Answer from the drawing. Dimensions are ordinates in mm from the lowest x, y and z of the part. A direction names the side the tool comes from. Give positions to 0.01 mm unless a question says otherwise; leave off trailing zeros. Loops run counter-clockwise (first coordinate to the right, second up) from the corner with the lowest first, then second, coordinate; pieces in that order, holes last. Notation, with made-up numbers: (16.5, 86) - (54.5, 86) arc R5 cw to (54.5, 92) - close; hole circle Ø2 at (-27, -14). An arc over 180 degrees is marked (long way). Answer as CSV lines item,"result". Start each with the question number.
1) A cutting plane is placed at D-D (z = 4.5). Determine the outline of the cut face in (x, y), and give its area (3 significant figures).
2) For a pull along X with two mould halves and no side action, classify the marked faces 3, 4, 5 and 6 as pulls with the +X half, pulls with the -X half, needs draft (parallel to the pull), parting line crosses it, or undercut.
3) A cutting plane is placed at B-B (x = 45.6). Determine the outline of the cut face in (y, z).
4) A cutting plane is placed at A-A (y = 21.4). Determine the outline of the cut face in (x, z).
5) A cutting plane is placed at C-C (y = 27). Determine the outline of the cut face in (x, z).
6) For the marked faces 1 and 2, determine the directions among +Z, -Z, +X, -X, +Y, -Y from which every point of the face is accessible in a straight line to the end or side of a thin tool.
7) Find the intervals of material crossed by line 1 along Y through (x, z) = (45.6, 10.8); line 2 along X through (y, z) = (8.5, 2.25); line 3 along Y through (x, z) = (19, 1.8), in increasing order.
8) Flat-ended cylindrical pins translate along their axes: pin 1 (2.5 mm diameter, centred on y = 23, z = 2, fed in from +X); pin 2 (1.7 mm diameter, centred on x = 2.4, y = 2.6, fed in from -Z); pin 3 (1.5 mm diameter, centred on x = 36, z = 6.5, fed in from +Y); pin 4 (6 mm diameter, centred on y = 32, z = 8, fed in from -X). Find the tip coordinate at first contact, or state that the pin passes through.
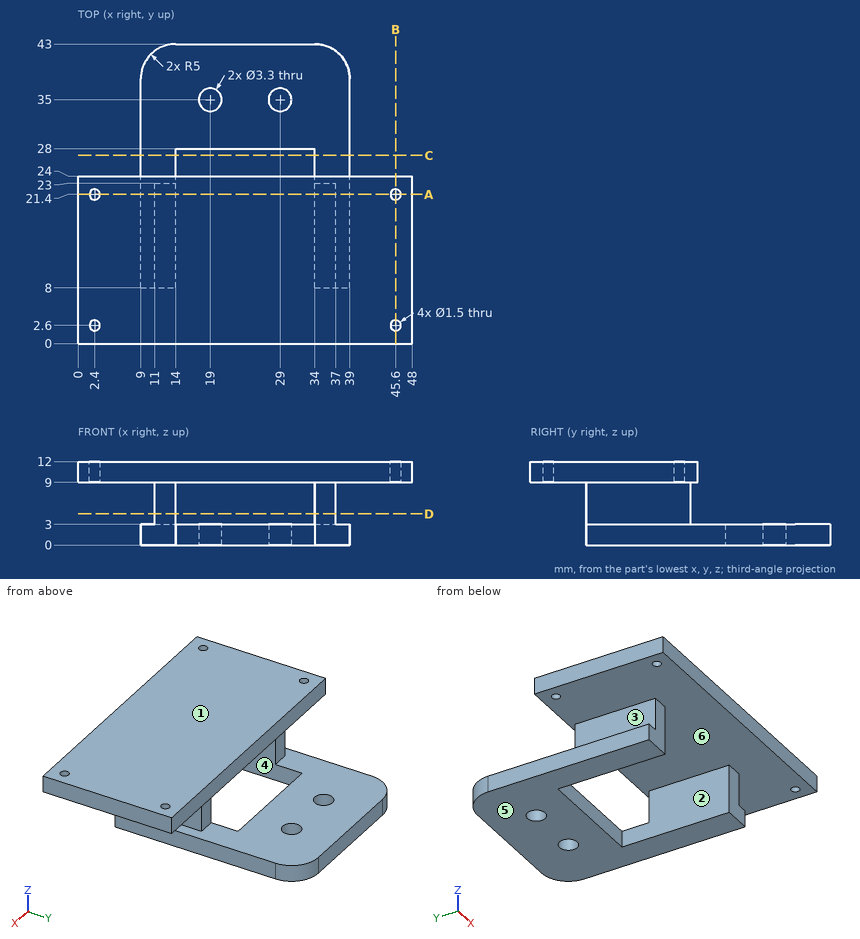
Ans:
1,outline,"(11, 8) - (14, 8) - (14, 23) - (11, 23) - close; (34, 8) - (37, 8) - (37, 23) - (34, 23) - close"
1,area,"90.0 mm2"
2,face 3,"pulls with the -X half"
2,face 4,"undercut"
2,face 5,"needs draft"
2,face 6,"undercut"
3,outline,"(0, 9) - (1.85, 9) - (1.85, 12) - (0, 12) - close; (3.35, 9) - (20.65, 9) - (20.65, 12) - (3.35, 12) - close; (22.15, 9) - (24, 9) - (24, 12) - (22.15, 12) - close"
4,outline,"(0, 9) - (1.65, 9) - (1.65, 12) - (0, 12) - close; (3.15, 9) - (11, 9) - (11, 3) - (9, 3) - (9, 0) - (14, 0) - (14, 9) - (34, 9) - (34, 0) - (39, 0) - (39, 3) - (37, 3) - (37, 9) - (44.85, 9) - (44.85, 12) - (3.15, 12) - close; (46.35, 9) - (48, 9) - (48, 12) - (46.35, 12) - close"
5,outline,"(9, 0) - (14, 0) - (14, 3) - (9, 3) - close; (34, 0) - (39, 0) - (39, 3) - (34, 3) - close"
6,face 1,"+Z, +X, -X, +Y, -Y"
6,face 2,"-Z, -Y"
7,line 1,"0 to 1.85, 3.35 to 20.65, 22.15 to 24"
7,line 2,"9 to 14, 34 to 39"
7,line 3,"28 to 33.35, 36.65 to 43"
8,pin 1,"x = 39"
8,pin 2,"z = 9"
8,pin 3,"y = 23"
8,pin 4,"through"
